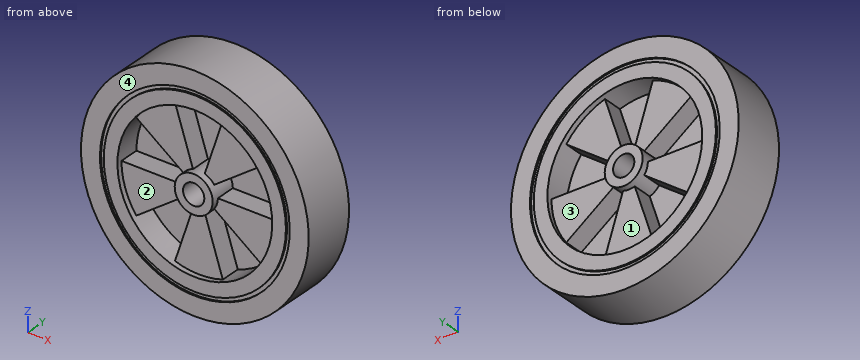
from build123d import *

# Parameters (mm, degrees)
SKETCH1_R           = 75
SKETCH1_R_2         = 51
BOSS_EXTRUDE1_DEPTH = 17.5
SKETCH2_R           = 12.5
SKETCH2_R_2         = 7
BOSS_EXTRUDE2_DEPTH = 18.5
BOSS_EXTRUDE3_DEPTH = 14
SKETCH6_R           = 51
BOSS_EXTRUDE6_DEPTH = 1
SKETCH7_R           = 62.5
SKETCH7_R_2         = 60
CUT_EXTRUDE1_DEPTH  = 1


with BuildPart() as part:
    # Sketch1 → Boss-Extrude1 (new, symmetric)
    with BuildSketch(Plane(origin=(0, 0, 0), x_dir=(1, 0, 0), z_dir=(0, 1, 0))):
        with Locations(Location((0, 0, 0), (0, 0, 270))):
            Circle(SKETCH1_R)
        with Locations(Location((0, 0, 0), (0, 0, 270))):
            Circle(SKETCH1_R_2, mode=Mode.SUBTRACT)
    extrude(amount=BOSS_EXTRUDE1_DEPTH, both=True)



with BuildPart() as body_2:
    # Sketch2 → Boss-Extrude2 (new, symmetric)
    with BuildSketch(Plane(origin=(0, 0, 0), x_dir=(1, 0, 0), z_dir=(0, 1, 0))):
        with Locations(Location((0, 0, 0), (0, 0, 270))):
            Circle(SKETCH2_R)
        with Locations(Location((0, 0, 0), (0, 0, 270))):
            Circle(SKETCH2_R_2, mode=Mode.SUBTRACT)
    extrude(amount=BOSS_EXTRUDE2_DEPTH, both=True)


with BuildPart() as part_1:
    add(part.part)

    add(body_2.part)  # Boss-Extrude3 merges body 2
    # Sketch3 → Boss-Extrude3 (add, symmetric)
    with BuildSketch(Plane(origin=(0, 0, 0), x_dir=(1, 0, 0), z_dir=(0, 1, 0))):
        with BuildLine():
            ThreePointArc((-12.5, 0), (-11.888206454, 3.86271243), (-10.11271243, 7.347315654))
            Line((-10.11271243, 7.347315654), (-41.259866713, 29.977047867))
            ThreePointArc((-41.259866713, 29.977047867), (-48.503882331, 15.759866713), (-51, 0))
            Line((-51, 0), (-12.5, 0))
        make_face()
        with BuildLine():
            ThreePointArc((-3.86271243, 11.888206454), (0, 12.5), (3.86271243, 11.888206454))
            Line((3.86271243, 11.888206454), (15.759866713, 48.503882331))
            ThreePointArc((15.759866713, 48.503882331), (0, 51), (-15.759866713, 48.503882331))
            Line((-15.759866713, 48.503882331), (-3.86271243, 11.888206454))
        make_face()
        with BuildLine():
            Line((41.259866713, 29.977047867), (10.11271243, 7.347315654))
            ThreePointArc((10.11271243, 7.347315654), (11.888206454, 3.86271243), (12.5, 0))
            Line((12.5, 0), (51, 0))
            ThreePointArc((51, 0), (48.503882331, 15.759866713), (41.259866713, 29.977047867))
        make_face()
        with BuildLine():
            Line((41.259866713, -29.977047867), (10.11271243, -7.347315654))
            ThreePointArc((10.11271243, -7.347315654), (7.347315654, -10.11271243), (3.86271243, -11.888206454))
            Line((3.86271243, -11.888206454), (15.759866713, -48.503882331))
            ThreePointArc((15.759866713, -48.503882331), (29.977047867, -41.259866713), (41.259866713, -29.977047867))
        make_face()
        with BuildLine():
            ThreePointArc((-3.86271243, -11.888206454), (-7.347315654, -10.11271243), (-10.11271243, -7.347315654))
            Line((-10.11271243, -7.347315654), (-41.259866713, -29.977047867))
            ThreePointArc((-41.259866713, -29.977047867), (-29.977047867, -41.259866713), (-15.759866713, -48.503882331))
            Line((-15.759866713, -48.503882331), (-3.86271243, -11.888206454))
        make_face()
    extrude(amount=BOSS_EXTRUDE3_DEPTH, both=True)

    # Sketch6 → Boss-Extrude6 (add, symmetric)
    with BuildSketch(Plane(origin=(0, 0, 0), x_dir=(1, 0, 0), z_dir=(0, 1, 0))):
        with Locations(Location((0, 0, 0), (0, 0, 72))):
            Circle(SKETCH6_R)
    extrude(amount=BOSS_EXTRUDE6_DEPTH, both=True)

    # Sketch7 → Cut-Extrude1 (cut)
    with BuildSketch(Plane(origin=(0, 17.5, 0), x_dir=(1, 0, 0), z_dir=(0, 1, 0))):
        with Locations(Location((0, 0, 0), (0, 0, 270))):
            Circle(SKETCH7_R)
        with Locations(Location((0, 0, 0), (0, 0, 270))):
            Circle(SKETCH7_R_2, mode=Mode.SUBTRACT)
    cut_extrude1 = extrude(amount=-CUT_EXTRUDE1_DEPTH, mode=Mode.SUBTRACT)

    # Mirror2: Cut-Extrude1 across plane
    add(cut_extrude1.mirror(Plane.ZX), mode=Mode.SUBTRACT)


solid = part_1.part
Could you check a few things on this model? Use its own coordinates, in mm. Face numbers are marked on the shaded views. A direction names the side the tool comes from. Coordinates: 2 decimals unless noted, no trailing zeros. Write each loop counter-clockwise with the first axis right and the second up, starting at its lowest first coordinate (ties: lowest second). Pieces come first, ordered by that corner, then holes. Notation, with made-up numbers: (25, 7) - (65, 7) arc R17 cw to (65, 13) - close; hole circle Ø4 at (9.5, -27.5). An arc over 180 degrees is marked (long way). Put each result on its own line as item: value. Start each with the question number.
Q1. Please list where these lines run through material, in increasing order: L1, parallel to X at y = 17, z = 0; L2, parallel to X at y = 16, z = 0; L3, parallel to Z at x = -40.5, y = -3.
Q2. I want a section at A-A on y = 10.5. Write out the boundary of the cut face in (x, z).
Q3. Thinking about a two-plate mould opening in Z: for the marked faces 3 and 4, which applies, pulls with the +Z half, pulls with the -Z half, needs draft (parallel to the pull), parting line crosses it, or undercut?
Q4. I'm going to push flat-ended pins straight in: P1, Ø8, axis at y = 13.5, z = 3.5, coming from the +X side; P2, Ø1.5, axis at x = 43.5, y = 9.5, coming from the -Z side; P3, Ø6, axis at x = 11, y = 9.5, coming from the -Z side; P4, Ø12, axis at x = -4.5, y = 6.5, coming from the +Z side. Where does each tip first touch, or does it pass through?
Q5. Which directions (+Z, -Z, +X, -X, +Y, -Y) give clear straight access to the entire face, cutting with the end or side of a thin tool? Please do the marked faces 1 and 2.
Q6. I want a section at B-B on x = 57. Write out the boundary of the cut face in (y, z) (3 decimals).
Checks:
1. L1: -75 to -62.5, -60 to -51, -12.5 to -7, 7 to 12.5, 51 to 60, 62.5 to 75
1. L2: -75 to -51, -12.5 to -7, 7 to 12.5, 51 to 75
1. L3: -63.12 to -31, -29.42 to 0, 29.42 to 63.12
2. outline: circle Ø150 at (0, 0); hole (-51, 0) - (-12.5, 0) arc R12.5 cw to (-10.11, 7.35) - (-41.26, 29.98) arc R51 ccw to start; hole (-41.26, -29.98) arc R51 ccw to (-15.76, -48.5) - (-3.86, -11.89) arc R12.5 cw to (-10.11, -7.35) - close; hole (-15.76, 48.5) - (-3.86, 11.89) arc R12.5 cw to (3.86, 11.89) - (15.76, 48.5) arc R51 ccw to start; hole circle Ø14 at (0, 0); hole (3.86, -11.89) - (15.76, -48.5) arc R51 ccw to (41.26, -29.98) - (10.11, -7.35) arc R12.5 cw to start; hole (10.11, 7.35) arc R12.5 cw to (12.5, 0) - (51, 0) arc R51 ccw to (41.26, 29.98) - close
3. face 3: undercut
3. face 4: needs draft
4. P1: x = 75
4. P2: z = -61.62
4. P3: z = -74.57
4. P4: z = 75
5. face 1: +Y
5. face 2: -Y
6. outline: (-17.5, -48.744) - (17.5, -48.744) - (17.5, -25.637) - (16.5, -25.637) - (16.5, -18.735) - (17.5, -18.735) - (17.5, 18.735) - (16.5, 18.735) - (16.5, 25.637) - (17.5, 25.637) - (17.5, 48.744) - (-17.5, 48.744) - (-17.5, 25.637) - (-16.5, 25.637) - (-16.5, 18.735) - (-17.5, 18.735) - (-17.5, -18.735) - (-16.5, -18.735) - (-16.5, -25.637) - (-17.5, -25.637) - close
